Verification items for this drawing (mm, ordinates from the low corner). A direction names the side the tool comes from. Round coordinates to 2 decimals unless told otherwise and drop trailing zeros. Loops run counter-clockwise (first coordinate to the right, second up) from the corner with the lowest first, then second, coordinate; pieces in that order, holes last. Notation, with made-up numbers: M 47.5,73 L 96.5,73 A19 ccw 96.5,93 Z; hole C 48.25,67.25 d1. An arc over 180 degrees is marked long. Write item = value, one per line.
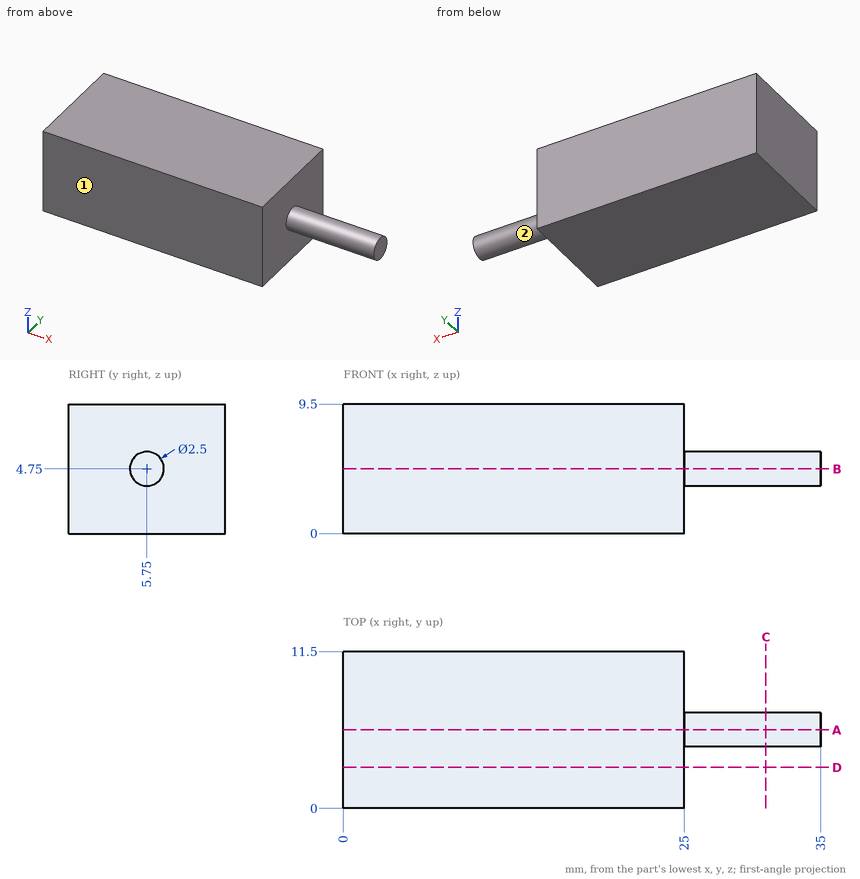
(1) Sectioned sample at A-A on y = 5.75. Record the cut outline in (x, z), then the cut area to 4 significant figures.
Result set:
outline = M 0,0 L 25,0 L 25,3.5 L 35,3.5 L 35,6 L 25,6 L 25,9.5 L 0,9.5 Z
area = 262.5 mm2
(2) Sectioned sample at D-D on y = 3. Record the cut outline in (x, z), then the cut area to 4 significant figures.
Result set:
outline = M 0,0 L 25,0 L 25,9.5 L 0,9.5 Z
area = 237.5 mm2
(3) Sectioned sample at C-C on x = 31. Record the cut outline in (y, z), then the cut area to 3 significant figures.
Result set:
outline = C 5.75,4.75 d2.5
area = 4.91 mm2
(4) Sectioned sample at B-B on z = 4.75. Record the cut outline in (x, y).
Result set:
outline = M 0,0 L 25,0 L 25,4.5 L 35,4.5 L 35,7 L 25,7 L 25,11.5 L 0,11.5 Z
(5) Tool access check on the marked faces 1 and 2. Record the directions out of +Z, -Z, +X, -X, +Y, -Y that give a thin tool (end or side, any length) a straight path to the whole face; none if there is none.
Result set:
face_1 = +Z, -Z, +X, -X, -Y
face_2 = +X
(6) Depth check by flat-ended pin: pin 1 Ø3 at (x, y) = (28, 6.5) entering from +Z. Enter the tip coordinate at first touch or a pass-through.
Result set:
pin_1 = 6
(7) Material ranges on line 1 along X through (y, z) = (2.25, 2.5); line 2 along Y through (x, z) = (32, 5); line 3 along Y through (x, z) = (31.5, 4), recorded low to high. Write a range as from..to.
Result set:
line_1 = 0..25
line_2 = 4.53..6.97
line_3 = 4.75..6.75
